CAD build for the part. Positions are in the model's coordinates, mm. A direction names the side the tool comes from. Coordinates: 2 decimals unless noted, no trailing zeros. Loops run counter-clockwise (first coordinate to the right, second up) from the corner with the lowest first, then second, coordinate; pieces in that order, holes last. Notation, with made-up numbers: (76.25, 15.5) - (131.25, 15.5) arc R18 ccw to (131.25, 39.5) - close; hole circle Ø10 at (74.5, 14). An arc over 180 degrees is marked (long way). Put each result on its own line as item: value.
```python
from build123d import *

# Parameters (mm, degrees)
ESQUISSE1_W      = 100
ESQUISSE1_H      = 130
ESQUISSE1_R      = 1.5
EXTRUSION1_DEPTH = 3
ESQUISSE2_W      = 55
ESQUISSE2_H      = 5
EXTRUSION2_DEPTH = 18
EXTRUSION3_DEPTH = 10
ESQUISSE4_W      = 10
ESQUISSE4_H      = 5
EXTRUSION4_DEPTH = 10


with BuildPart() as part:
    # Esquisse1 → Extrusion1 (new body)
    with BuildSketch(Plane(origin=(0, 0, 0), x_dir=(1, 0, 0), z_dir=(0, 1, 0))):
        with Locations((50, 65)):
            Rectangle(ESQUISSE1_W, ESQUISSE1_H)
        with Locations((5, 125)):
            Circle(ESQUISSE1_R, mode=Mode.SUBTRACT)
        with Locations((95, 125)):
            Circle(ESQUISSE1_R, mode=Mode.SUBTRACT)
        with Locations((95, 5)):
            Circle(ESQUISSE1_R, mode=Mode.SUBTRACT)
        with Locations((5, 5)):
            Circle(ESQUISSE1_R, mode=Mode.SUBTRACT)
    extrude(amount=EXTRUSION1_DEPTH)

    # Esquisse2 → Extrusion2 (add)
    with BuildSketch(Plane(origin=(0, 3, 0), x_dir=(1, 0, 0), z_dir=(0, 1, 0))):
        with Locations((54.5, 105.5)):
            Rectangle(ESQUISSE2_W, ESQUISSE2_H)
        with Locations((54.5, 35.5)):
            Rectangle(ESQUISSE2_W, ESQUISSE2_H)
    extrude(amount=EXTRUSION2_DEPTH)

    # Esquisse3 → Extrusion3 (add)
    with BuildSketch(Plane(origin=(0, 3, 0), x_dir=(1, 0, 0), z_dir=(0, 1, 0))):
        Polygon((22.725382584, 0), (22.725382584, 10), (52.725382584, 10), (52.725382584, 0), (47.725382584, 0), (47.725382584, -10), (27.725382584, -10), (27.725382584, 0), align=None)
    extrude(amount=EXTRUSION3_DEPTH)

    # Esquisse4 → Extrusion4 (add)
    with BuildSketch(Plane(origin=(0, 3, 0), x_dir=(1, 0, 0), z_dir=(0, 1, 0))):
        with Locations((22.654691777, 123.012698359)):
            Rectangle(ESQUISSE4_W, ESQUISSE4_H)
        with Locations((40.154691777, 123.012698359)):
            Rectangle(ESQUISSE4_W, ESQUISSE4_H)
        with Locations((57.654691777, 123.012698359)):
            Rectangle(ESQUISSE4_W, ESQUISSE4_H)
        with Locations((75.154691777, 123.012698359)):
            Rectangle(ESQUISSE4_W, ESQUISSE4_H)
    extrude(amount=EXTRUSION4_DEPTH)


solid = part.part
```
Q1. Pin check, flat tips, straight feed: pin 1 Ø1.5 at (y, z) = (8.5, -124) entering from +X; pin 2 Ø5 at (x, z) = (5, -125) entering from +Y; pin 3 Ø8 at (y, z) = (10, -6.5) entering from -X. Stop position of each tip, or through.
Determined:
pin 1: x = 80.15
pin 2: y = 3
pin 3: x = 22.73
Q2. Slice it at D-D, the plane y = 16.25. Give the cut face in (x, z), then the cut area to 3 significant figures.
Determined:
outline: (27, -108) - (82, -108) - (82, -103) - (27, -103) - close; (27, -38) - (82, -38) - (82, -33) - (27, -33) - close
area: 550 mm2
Q3. Tool access for faces 1 (the flat face through (82, 12, -35)), 2 (the flat face through (58, 8, -120.513)), 3 (the flat face through (75, 13, -123)): list every direction of +Z, -Z, +X, -X, +Y, -Y with a clear straight run to the whole face (end or side of a thin tool).
Determined:
face 1: +Z, -Z, +X, +Y
face 2: +X, -X, +Y
face 3: -Z, +X, -X, +Y
Q4. Mould opens along X. For faces 4 (the flat face through (52.655, 8, -123)), 5 (the flat face through (38, 8, -10)), 6 (the flat face through (22.725, 8, -5)) say: +X half, -X half, draft (parallel to the pull), parting line (faces both ways), or undercut.
Determined:
face 4: undercut
face 5: draft
face 6: -X half
Q5. Slice it at C-C, the plane x = 95. Give the cut face in (y, z).
Determined:
outline: (0, -130) - (3, -130) - (3, -126.5) - (0, -126.5) - close; (0, -123.5) - (3, -123.5) - (3, -6.5) - (0, -6.5) - close; (0, -3.5) - (3, -3.5) - (3, 0) - (0, 0) - close
Q6. Slice it at A-A, the plane y = 5.5. State how many separate pieces and enclosed holes the cut face has, then the cut area to 3 significant figures.
Determined:
separate pieces: 7
enclosed holes: 0
area: 1,250 mm2
Q7. Slice it at B-B, the plane z = -5. Give the cut face in (x, y).
Determined:
outline: (0, 0) - (3.5, 0) - (3.5, 3) - (0, 3) - close; (6.5, 0) - (93.5, 0) - (93.5, 3) - (52.73, 3) - (52.73, 13) - (22.73, 13) - (22.73, 3) - (6.5, 3) - close; (96.5, 0) - (100, 0) - (100, 3) - (96.5, 3) - close
Q8. Wall check: L1, parallel to X at y = 1.7, z = -125; L2, parallel to Z at x = 77, y = 8.5; L3, parallel to Z at x = 5, y = 1.7. Give the ranges that are in metal, low to high. Write a range as from..to.
Determined:
L1: 0..3.5, 6.5..93.5, 96.5..100
L2: -125.51..-120.51, -108..-103, -38..-33
L3: -130..-126.5, -123.5..-6.5, -3.5..0
